```python
from build123d import *

# Parameters (mm, degrees)
SKETCH1_R           = 82.832169861
BOSS_EXTRUDE1_DEPTH = 5
SKETCH3_W           = 93.167206873
SKETCH3_H           = 4.120105984
CUT_EXTRUDE1_DEPTH  = 75
SKETCH4_R           = 27.598349682
SKETCH4_R_2         = 22.972927947
CUT_EXTRUDE2_DEPTH  = 1
BOSS_EXTRUDE2_START = 11
SKETCH5_R           = 77.433591729
BOSS_EXTRUDE2_DEPTH = 11
FILLET1_R           = 10
SKETCH6_W           = 49.330343736
SKETCH6_H           = 20
BOSS_EXTRUDE3_DEPTH = 46
CUT_EXTRUDE3_DEPTH  = 46
CIRPATTERN1_COUNT   = 4


with BuildPart() as part:
    # Sketch1 → Boss-Extrude1 (new body)
    with BuildSketch(Plane(origin=(0, 0, 0), x_dir=(1, 0, 0), z_dir=(0, 1, 0))):
        with Locations(Location((-49.943747887, -23.441982102, 0), (0, 0, 270))):
            Circle(SKETCH1_R)
        with BuildLine():
            Line((-59.943747887, 50.888361635), (-59.943747887, 1.558017898))
            Line((-59.943747887, 1.558017898), (-39.943747887, 1.558017898))
            Line((-39.943747887, 1.558017898), (-39.943747887, 50.888361635))
            ThreePointArc((-39.943747887, 50.888361635), (3.089260702, 29.591026487), (24.386595849, -13.441982102))
            Line((24.386595849, -13.441982102), (-24.943747887, -13.441982102))
            Line((-24.943747887, -13.441982102), (-24.943747887, -33.441982102))
            Line((-24.943747887, -33.441982102), (24.386595849, -33.441982102))
            ThreePointArc((24.386595849, -33.441982102), (3.089260702, -76.474990691), (-39.943747887, -97.772325838))
            Line((-39.943747887, -97.772325838), (-39.943747887, -48.441982102))
            Line((-39.943747887, -48.441982102), (-59.943747887, -48.441982102))
            Line((-59.943747887, -48.441982102), (-59.943747887, -97.772325838))
            ThreePointArc((-59.943747887, -97.772325838), (-102.976756476, -76.474990691), (-124.274091624, -33.441982102))
            Line((-124.274091624, -33.441982102), (-74.943747887, -33.441982102))
            Line((-74.943747887, -33.441982102), (-74.943747887, -13.441982102))
            Line((-74.943747887, -13.441982102), (-124.274091624, -13.441982102))
            ThreePointArc((-124.274091624, -13.441982102), (-102.976756476, 29.591026487), (-59.943747887, 50.888361635))
        make_face(mode=Mode.SUBTRACT)
    extrude(amount=BOSS_EXTRUDE1_DEPTH)

    # Sketch2 → Revolve1 (revolve)
    with BuildSketch(Plane.XY.offset(23.441982102)):
        with BuildLine():
            Line((-49.943747887, 5), (-49.943747887, 25.910941369))
            add(Edge.make_bspline(
                [(32.888421974, 5), (32.888421974, 25.910941369), (-49.943747887, 25.910941369)],
                knots=[0, 0, 0, 1.570796327, 1.570796327, 1.570796327], degree=2, weights=[1, 0.707106781, 1]))
            Line((32.888421974, 5), (-49.943747887, 5))
        make_face()
    revolve(axis=Axis((-49.943747887, 5, 23.441982102), (0, 1, 0)))

    # Sketch3 → Cut-Extrude1 (cut, symmetric)
    with BuildSketch(Plane.XY.offset(23.441982102)):
        with Locations((-49.943747888, 25.910941369)):
            Rectangle(SKETCH3_W, SKETCH3_H)
    extrude(amount=CUT_EXTRUDE1_DEPTH, both=True, mode=Mode.SUBTRACT)

    # Sketch4 → Cut-Extrude2 (cut)
    with BuildSketch(Plane(origin=(0, 23.850888377, 0), x_dir=(1, 0, 0), z_dir=(0, 1, 0))):
        with Locations(Location((-49.943747887, -23.441982102, 0), (0, 0, 270))):
            Circle(SKETCH4_R)
        with Locations(Location((-49.943747887, -23.441982102, 0), (0, 0, 270))):
            Circle(SKETCH4_R_2, mode=Mode.SUBTRACT)
    extrude(amount=-CUT_EXTRUDE2_DEPTH, mode=Mode.SUBTRACT)

    # Sketch5 → Boss-Extrude2 (add)
    with BuildSketch(Plane.XZ.offset(BOSS_EXTRUDE2_START)):
        with Locations(Location((-49.943747887, 23.441982102, 0), (0, 0, 90))):
            Circle(SKETCH5_R)
        with BuildLine():
            Line((-59.943747887, 97.772325838), (-59.943747887, 48.441982102))
            Line((-59.943747887, 48.441982102), (-39.943747887, 48.441982102))
            Line((-39.943747887, 48.441982102), (-39.943747887, 97.772325838))
            ThreePointArc((-39.943747887, 97.772325838), (3.089260702, 76.474990691), (24.386595849, 33.441982102))
            Line((24.386595849, 33.441982102), (-24.943747887, 33.441982102))
            Line((-24.943747887, 33.441982102), (-24.943747887, 13.441982102))
            Line((-24.943747887, 13.441982102), (24.386595849, 13.441982102))
            ThreePointArc((24.386595849, 13.441982102), (3.089260702, -29.591026487), (-39.943747887, -50.888361635))
            Line((-39.943747887, -50.888361635), (-39.943747887, -1.558017898))
            Line((-39.943747887, -1.558017898), (-59.943747887, -1.558017898))
            Line((-59.943747887, -1.558017898), (-59.943747887, -50.888361635))
            ThreePointArc((-59.943747887, -50.888361635), (-102.976756476, -29.591026487), (-124.274091624, 13.441982102))
            Line((-124.274091624, 13.441982102), (-74.943747887, 13.441982102))
            Line((-74.943747887, 13.441982102), (-74.943747887, 33.441982102))
            Line((-74.943747887, 33.441982102), (-124.274091624, 33.441982102))
            ThreePointArc((-124.274091624, 33.441982102), (-102.976756476, 76.474990691), (-59.943747887, 97.772325838))
        make_face(mode=Mode.SUBTRACT)
    extrude(amount=-BOSS_EXTRUDE2_DEPTH)

    # Fillet1
    # the kernel refuses this fillet: 10 mm, written as the material it adds along each edge
    with BuildSketch(Plane(origin=(-49.943747887, 0, 23.441982102), x_dir=(0, 0, 1), z_dir=(1, 0, 0))) as fillet1_piece_1:
        with BuildLine():
            CenterArc((87.433591729, 8.878452387), FILLET1_R, 180, 62.603717063)
            Line((77.433591729, 8.878452387), (77.233591729, 8.878452387))
            Line((77.233591729, 8.878452387), (77.233591729, 0))
            Line((77.233591729, 0), (77.433591729, -0.2))
            ThreePointArc((77.433591729, -0.2), (80.132880795, -0.2), (82.740141424, -0.177569048))
            Line((82.740141424, -0.177569048), (82.832169861, 0))
        make_face()
    revolve(axis=Axis((-49.943747887, 0, 23.441982102), (0, -1, 0)))

    # Sketch6 → Boss-Extrude3 (add)
    with BuildSketch(Plane.XZ.offset(11)):
        with Locations((-0.278576019, 23.441982102)):
            Rectangle(SKETCH6_W, SKETCH6_H)
    boss_extrude3 = extrude(amount=BOSS_EXTRUDE3_DEPTH)

    # Sketch7 → Cut-Extrude3 (cut)
    with BuildSketch(Plane.XY.offset(33.441982102)):
        Polygon((24.386595849, -11), (-24.943747887, -57), (24.386595849, -57), align=None)
    cut_extrude3 = extrude(amount=-CUT_EXTRUDE3_DEPTH, mode=Mode.SUBTRACT)

    # CirPattern1: Boss-Extrude3, Cut-Extrude3 ×4 about axis
    cirpattern1_axis = Axis((-49.943747887, 0, 23.441982102), (0, 1, 0))
    add([boss_extrude3.rotate(cirpattern1_axis, i * 360 / CIRPATTERN1_COUNT) for i in range(1, CIRPATTERN1_COUNT)])
    add([cut_extrude3.rotate(cirpattern1_axis, i * 360 / CIRPATTERN1_COUNT) for i in range(1, CIRPATTERN1_COUNT)], mode=Mode.SUBTRACT)


solid = part.part
```
Verification items for the finished model (mm, model axes). A direction names the side the tool comes from. Round coordinates to 2 decimals unless told otherwise and drop trailing zeros. Write each loop counter-clockwise with the first axis right and the second up, starting at its lowest first coordinate (ties: lowest second). Pieces come first, ordered by that corner, then holes.
1. Access from +Z, -Z, +X, -X, +Y, -Y to the whole of each face (thin tool, end or side, straight path). Record for faces 5 (the flat face through (-29, 22.851, 13)), 6 (the flat face through (-32, 23.851, 2)), 7 (the flat face through (-59.944, -19, -20)).
2. Section check A-A on y = -29. Enter the section's corners in (x, z), plus the area to 3 significant figures.
3. Draft check along Z on faces 1 (the flat face through (-50, -26, -1.558)), 2 (the cylindrical face through (-102.277, -9.954, -33.63)), 3 (the flat face through (-113.4, -11, -17.1)), 4 (the flat face through (-50, -26, 48.442)). Enter one of: +Z half, -Z half, draft (parallel to the pull), parting line (faces both ways), or undercut.
4. Gauge pin test, flat ends, axial feed: P1, Ø2, axis at x = 11.5, z = 1.5, coming from the +Y side; P2, Ø3, axis at x = -31.5, y = 10, coming from the -Z side; P3, Ø2, axis at y = -3, z = -18, coming from the -X side. Record the tip position at first contact, or that the pin passes through.
5. Scan lines: L1, parallel to X at y = 3, z = 78.5; L2, parallel to Y at x = -71, z = 61; L3, parallel to X at y = -11.5, z = -39. Record each from-to range of solid material in increasing order.
6. Section check B-B on y = -46.5. Enter the section's corners in (x, z).
Answer:
1. face 5: +Y
1. face 6: +Z, -Z, +X, -X, +Y
1. face 7: -Y
2. outline: (-104.97, 13.44) - (-74.94, 13.44) - (-74.94, 33.44) - (-104.97, 33.44) - close; (-59.94, -31.59) - (-39.94, -31.59) - (-39.94, -1.56) - (-59.94, -1.56) - close; (-59.94, 48.44) - (-39.94, 48.44) - (-39.94, 78.47) - (-59.94, 78.47) - close; (-24.94, 13.44) - (5.08, 13.44) - (5.08, 33.44) - (-24.94, 33.44) - close
2. area: 2,400 mm2
3. face 1: undercut
3. face 2: parting line
3. face 3: draft
3. face 4: undercut
4. P1: stops at y = 18.2
4. P2: stops at z = -56.17
4. P3: stops at x = -118.73
5. L1: x = -111.83 to -100.87, -59.94 to -39.94, 0.98 to 11.94
5. L2: y = 5 to 22.86
5. L3: x = -59.94 to -39.94
6. outline: (-86.2, 13.44) - (-74.94, 13.44) - (-74.94, 33.44) - (-86.2, 33.44) - close; (-59.94, -12.82) - (-39.94, -12.82) - (-39.94, -1.56) - (-59.94, -1.56) - close; (-59.94, 48.44) - (-39.94, 48.44) - (-39.94, 59.7) - (-59.94, 59.7) - close; (-24.94, 13.44) - (-13.68, 13.44) - (-13.68, 33.44) - (-24.94, 33.44) - close
